Source: CAD feature listing. Evaluate the final solid. Frame: model axes, mm. Face numbers are marked on the shaded views. A direction names the side the tool comes from. Round coordinates to 2 decimals unless told otherwise and drop trailing zeros. Write each loop counter-clockwise with the first axis right and the second up, starting at its lowest first coordinate (ties: lowest second). Pieces come first, ordered by that corner, then holes. Notation, with made-up numbers: M -2.5,-5.5 L 3.5,-5.5 A24 ccw 3.5,29.5 Z; hole C -2,31.5 d3. An arc over 180 degrees is marked long. Answer in a Markdown table with one row per item. Add a question column.
Item 1: Cut plane B-B on x = 0. Return loops of the section in (y, z), and give its area (3 significant figures).
Item 2: Cut plane A-A on z = 0. Return loops of the section in (x, y).
Item 3: Cut plane D-D on z = 0.55. Return loops of the section in (x, y).
Item 4: Contact query for flat-ended pins moving along their axis: pin 1 (1.2 mm diameter, centred on x = 1, z = 1.5, fed in from +Y); pin 2 (2 mm diameter, centred on y = 2.5, z = 1, fed in from +X); pin 3 (1.5 mm diameter, centred on x = 1, z = 1, fed in from +Y). Output: stop coordinate, or through.
Item 5: Mould query, pull axis Z, two halves, no side actions, for the marked faces 6, 7 and 8. Classes: released by +Z, released by -Z, zero draft, split by the parting line, or undercut.
Item 6: Set-up query: the marked faces 1, 2, 3, 4 and 5. Return all of +Z, -Z, +X, -X, +Y, -Y with unobstructed straight access to the full face (end or side cutting, diameter ignored); none if empty.
Item 7: Cut plane C-C on y = 3.75. Return loops of the section in (x, z), and give its area (3 significant figures).
Item 8: Material intervals for probe 1 along X at (y, z) = (4.5, 0); probe 2 along Z at (x, y) = (0.1, 1); probe 3 along Z at (x, y) = (-0.45, 5), sorted ascending.
from build123d import *

# Parameters (mm, degrees)
SKETCH_4_R          = 1.6
CUT_EXTRUDE_1_DEPTH = 6
SKETCH_5_W          = 6.845786851
SKETCH_5_H          = 1.5
CUT_EXTRUDE_3_DEPTH = 3


with BuildPart() as part:
    # 草图3 → 旋转1 (revolve)
    with BuildSketch(Plane(origin=(0, 0, 0), x_dir=(0, 0, -1), z_dir=(1, 0, 0)), mode=Mode.PRIVATE) as revolve_1_sk:
        with BuildLine():
            Line((2.4, 6.791402502), (2.4, 6))
            Line((2.4, 6), (2, 6))
            Line((2, 6), (2, 2.5))
            Line((2, 2.5), (2.2, 2.5))
            ThreePointArc((2.2, 2.5), (2.341421356, 2.441421356), (2.4, 2.3))
            Line((2.4, 2.3), (2.4, 1))
            ThreePointArc((2.4, 1), (2.107106781, 0.292893219), (1.4, 0))
            Line((1.4, 0), (0, 0))
            Line((0, 0), (0, 7.5))
            ThreePointArc((0, 7.5), (1.251210455, 7.319149638), (2.4, 6.791402502))
        make_face()
    revolve(revolve_1_sk.sketch.rotate(Axis((0, 28.211895781, 0), (0, -1, 0)), 180), axis=Axis((0, 28.211895781, 0), (0, -1, 0)))

    # 草图4 → 切除-拉伸1 (cut)
    with BuildSketch(Plane.XZ):
        with Locations(Location((0, 0, 0), (0, 0, 270))):
            Circle(SKETCH_4_R)
    extrude(amount=-CUT_EXTRUDE_1_DEPTH, mode=Mode.SUBTRACT)

    # 草图5 → 切除-拉伸3 (cut)
    with BuildSketch(Plane(origin=(0, 0, 0), x_dir=(1, 0, 0), z_dir=(0, 1, 0))):
        with Locations((0.068457868, 0)):
            Rectangle(SKETCH_5_W, SKETCH_5_H)
    extrude(amount=CUT_EXTRUDE_3_DEPTH, mode=Mode.SUBTRACT)


solid = part.part
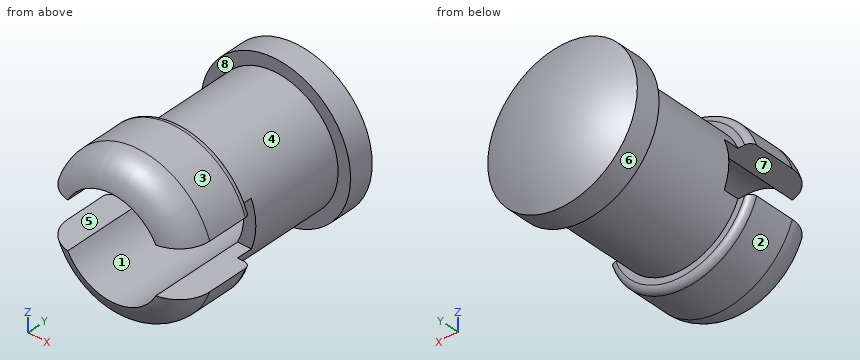
Results below:
| question | item | result |
|---|---|---|
| 1 | outline | M 0.02,-1.6 A1 ccw 1,-2.4 L 2.3,-2.4 A0.2 ccw 2.5,-2.2 L 2.5,-2 L 6,-2 L 6,-2.4 L 6.79,-2.4 A4.42 ccw 6.79,2.4 L 6,2.4 L 6,2 L 2.5,2 L 2.5,2.2 A0.2 ccw 2.3,2.4 L 1,2.4 A1 ccw 0.02,1.6 L 6,1.6 L 6,-1.6 Z |
| 1 | area | 12.5 mm2 |
| 2 | outline | M -2.4,6 L -2,6 L -2,3 L -1.6,3 L -1.6,6 L 1.6,6 L 1.6,3 L 2,3 L 2,6 L 2.4,6 L 2.4,6.79 A4.42 ccw -2.4,6.79 Z |
| 3 | outline | M -2.34,6 L -1.92,6 L -1.92,3 L -1.5,3 L -1.5,6 L 1.5,6 L 1.5,3 L 1.92,3 L 1.92,6 L 2.34,6 L 2.34,6.79 A4.38 ccw -2.34,6.79 Z |
| 4 | pin 1 | y = 7.33 |
| 4 | pin 2 | x = 2.28 |
| 4 | pin 3 | y = 7.45 |
| 5 | face 6 | split by the parting line |
| 5 | face 7 | undercut |
| 5 | face 8 | zero draft |
| 6 | face 1 | -Y |
| 6 | face 2 | -Z, +Y, -Y |
| 6 | face 3 | +Z, +Y, -Y |
| 6 | face 4 | none |
| 6 | face 5 | +X, -X, -Y |
| 7 | outline | C 0,0 d4; hole C 0,0 d3.2 |
| 7 | area | 4.52 mm2 |
| 8 | probe 1 | -2 to -1.6, 1.6 to 2 |
| 8 | probe 2 | -2.4 to -1.6, 1.6 to 2.4 |
| 8 | probe 3 | -1.95 to -1.54, 1.54 to 1.95 |
